Geometry check sheet. Reference: drawing and pictorial views, mm from the part's lowest x, y, z. Give positions to 0.01 mm unless a question says otherwise; leave off trailing zeros. Write each loop counter-clockwise with the first axis right and the second up, starting at its lowest first coordinate (ties: lowest second). Pieces come first, ordered by that corner, then holes. Notation, with made-up numbers: (38, 58.5) -> (87, 58.5) arc R32 cw to (87, 96.5) -> close; hole circle Ø5 at (88.5, -1). An arc over 180 degrees is marked (long way). Return JSON: item names as keys, results as strings.
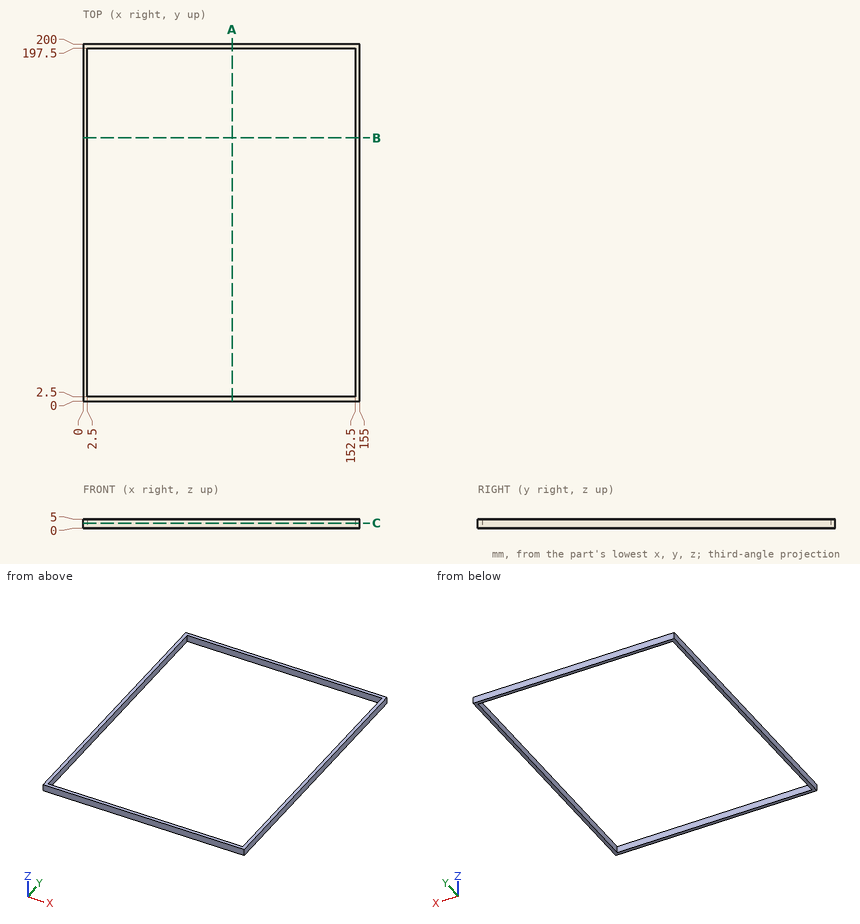
(1) Cross-section at A-A on x = 83.5. Enter the section's corners in (y, z).
Reply:
{"outline": "(0, 0) -> (2.5, 0) -> (2.5, 5) -> (0, 5) -> close; (197.5, 0) -> (200, 0) -> (200, 5) -> (197.5, 5) -> close"}
(2) Thickness scan on L1, parallel to X at y = 164, z = 0.4; L2, parallel to Y at x = 105, z = 1.6. Record the ranges inside material, lowest first.
Reply:
{"L1": "0 to 2.5, 152.5 to 155", "L2": "0 to 2.5, 197.5 to 200"}
(3) Cross-section at C-C on z = 2.75. Enter the section's corners in (x, y).
Reply:
{"outline": "(0, 0) -> (155, 0) -> (155, 200) -> (0, 200) -> close; hole (2.5, 2.5) -> (152.5, 2.5) -> (152.5, 197.5) -> (2.5, 197.5) -> close"}
(4) Cross-section at B-B on y = 147.5. Enter the section's corners in (x, z).
Reply:
{"outline": "(0, 0) -> (2.5, 0) -> (2.5, 5) -> (0, 5) -> close; (152.5, 0) -> (155, 0) -> (155, 5) -> (152.5, 5) -> close"}
